Geometry check sheet. Reference: the model listing, model coordinates, mm. Face numbers are marked on the shaded views. A direction names the side the tool comes from. Round coordinates to 2 decimals unless told otherwise and drop trailing zeros. Order: outer loops, then holes, each group sorted by start corner. A loop starts at its lowest first (then second) coordinate and runs counter-clockwise, first axis right, second up.
(1) Release check for a two-part mould opening along Z. For the marked faces 1, 2 and 3 record: +Z half, -Z half, draft (parallel to the pull), parting line (faces both ways), or undercut.
(2) Go/stop test with flat-tipped pins: pin 1 (6 mm diameter, centred on x = -55.5, z = -14.5, fed in from +Y); pin 2 (4 mm diameter, centred on x = -86, y = -161, fed in from -Z); pin 3 (8 mm diameter, centred on y = -143, z = -8.5, fed in from -X); pin 4 (1 mm diameter, centred on y = -146, z = -13.5, fed in from -X). Record where each tip stops, or that it passes through.
(3) Sectioned sample at D-D (z = -3). Record the boundary of the cut face in (x, y), plus the area to 3 significant figures.
(4) Sectioned sample at B-B (x = -46). Record the boundary of the cut face in (y, z), plus the area to 3 significant figures.
(5) Material ranges on line 1 along Z through (x, y) = (-58, -156.5); line 2 along Y through (x, z) = (-63, -15.25); line 3 along X through (y, z) = (-153.25, -11), recorded low to high.
(6) Sectioned sample at A-A (y = -158.5). Record the boundary of the cut face in (x, z), plus the area to 3 significant figures.
(7) Sectioned sample at C-C (y = -151.5). Record the boundary of the cut face in (x, z), plus the area to 3 significant figures.
(8) Set-up check for the marked faces 4 and 5: record each of +Z, -Z, +X, -X, +Y, -Y from which the full face is reachable in a straight line by a thin tool's end or side.
from build123d import *

# Parameters (mm, degrees)
ESBO_O1_R                = 3
RESSALTO_EXTRUS_O1_DEPTH = 2
RESSALTO_EXTRUS_O2_DEPTH = 13
CORTE_EXTRUS_O1_REACH    = 100.627
ESBO_O7_R                = 2.5
CORTE_EXTRUS_O2_REACH    = 98.131
ESBO_O6_R                = 2.5


with BuildPart() as part:
    # Esboço1 → Ressalto-extrusão1 (new body)
    with BuildSketch(Plane.XY):
        Polygon((-42.366282029, -174), (-42.366282029, -154.146561088), (-63.935449693, -154.146561088), (-79.437349841, -138.644660941), (-93.579485465, -152.786796564), (-85.828535391, -160.537746638), (-78.077585317, -168.288696712), (-72.366282029, -174), align=None)
        with Locations((-53.150865861, -164.073280544)):
            Circle(ESBO_O1_R, mode=Mode.SUBTRACT)
        with Locations((-78.757467579, -153.466678826)):
            Circle(ESBO_O1_R, mode=Mode.SUBTRACT)
    ressalto_extrus_o1 = extrude(amount=RESSALTO_EXTRUS_O1_DEPTH)

    # Esboço5 → Ressalto-extrusão2 (add)
    with BuildSketch(Plane.XY.offset(2)):
        Polygon((-78.376689669, -137.290878593), (-79.437349841, -138.644660941), (-63.935449693, -154.146561088), (-42.366282029, -154.146561088), (-42.366282029, -152.5), (-63.167568262, -152.5), align=None)
    ressalto_extrus_o2 = extrude(amount=-RESSALTO_EXTRUS_O2_DEPTH)

    # Espelhar2: Ressalto-extrusão1, Ressalto-extrusão2 across plane
    add(ressalto_extrus_o1.mirror(Plane.XY.offset(-11)))
    add(ressalto_extrus_o2.mirror(Plane.XY.offset(-11)))

    # Esboço7 → Corte-extrusão1 (cut, up to next)
    with BuildSketch(Plane.XZ.offset(154.146561088), mode=Mode.PRIVATE) as corte_extrus_o1_sk1:
        with Locations(Location((-53.150865861, -11, 0), (0, 0, 270))):
            Circle(ESBO_O7_R)
    corte_extrus_o1_tool1 = extrude(corte_extrus_o1_sk1.sketch, amount=-CORTE_EXTRUS_O1_REACH, mode=Mode.PRIVATE) & part.part
    add(corte_extrus_o1_tool1.solids().sort_by_distance((-53.150866, -154.146561, -11))[0], mode=Mode.SUBTRACT)

    # Esboço6 → Corte-extrusão2 (cut, up to next)
    with BuildSketch(Plane(origin=(-109.041005391, -109.041005391, 0), x_dir=(-0.7071067811865478, 0.7071067811865472, 0), z_dir=(-0.7071067811865472, -0.7071067811865478, 0)), mode=Mode.PRIVATE) as corte_extrus_o2_sk1:
        with Locations(Location((-52.82738989, 11, 0), (0, 0, 180))):
            Circle(ESBO_O6_R)
    corte_extrus_o2_tool1 = extrude(corte_extrus_o2_sk1.sketch, amount=-CORTE_EXTRUS_O2_REACH, mode=Mode.PRIVATE) & part.part
    add(corte_extrus_o2_tool1.solids().sort_by_distance((-71.6864, -146.395611, -11))[0], mode=Mode.SUBTRACT)


solid = part.part
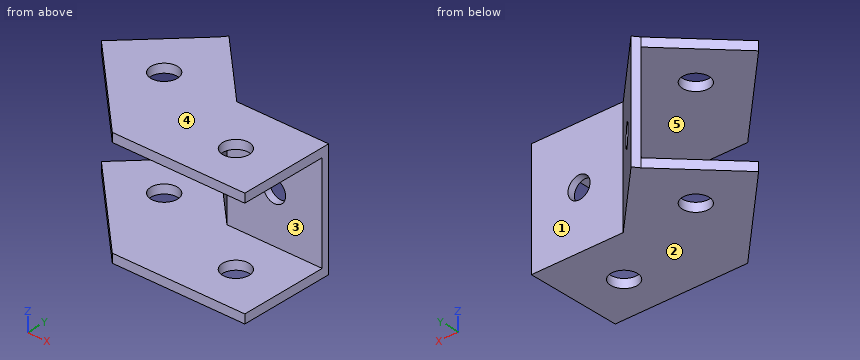
Answer below:
1. face 1: draft
1. face 2: -Z half
1. face 3: undercut
2. pin 1: stops at y = -152.5
2. pin 2: stops at z = -24
2. pin 3: stops at x = -79.08
2. pin 4: stops at x = -72.58
3. outline: (-79.44, -138.64) - (-63.94, -154.15) - (-42.37, -154.15) - (-42.37, -152.5) - (-63.17, -152.5) - (-78.38, -137.29) - close
3. area: 72.0 mm2
4. outline: (-174, -24) - (-152.5, -24) - (-152.5, 2) - (-174, 2) - (-174, 0) - (-154.15, 0) - (-154.15, -22) - (-174, -22) - close
4. area: 122 mm2
5. line 1: z = -24 to -22, 0 to 2
5. line 2: y = -154.15 to -152.5
5. line 3: x = -64.83 to -55.65, -50.65 to -42.37
6. outline: (-87.87, -24) - (-42.37, -24) - (-42.37, -22) - (-87.87, -22) - close; (-87.87, 0) - (-42.37, 0) - (-42.37, 2) - (-87.87, 2) - close
6. area: 182 mm2
7. outline: (-92.29, -24) - (-81.02, -24) - (-81.02, -22) - (-92.29, -22) - close; (-92.29, 0) - (-81.02, 0) - (-81.02, 2) - (-92.29, 2) - close; (-76.49, -24) - (-64.17, -24) - (-64.17, 2) - (-76.49, 2) - (-76.49, 0) - (-66.58, 0) - (-66.58, -22) - (-76.49, -22) - close
7. area: 147 mm2
8. face 4: +Z, +X, -X, +Y, -Y
8. face 5: -X, -Y
